```python
from build123d import *

# Parameters (mm, degrees)
BOSS_EXTRUDE1_DEPTH = 10.52068
BOSS_EXTRUDE3_DEPTH = 5.588
SKETCH4_R           = 1.037113256
CUT_EXTRUDE1_DEPTH  = 5.588
SKETCH5_R           = 0.970454713
CUT_EXTRUDE2_DEPTH  = 10.52068


with BuildPart() as part:
    # Sketch1 → Boss-Extrude1 (new body)
    with BuildSketch(Plane(origin=(0, 0, 0), x_dir=(0, 0, -1), z_dir=(1, 0, 0))):
        with BuildLine():
            Line((0, 0), (0, 5.588000005))
            add(Edge.make_bspline(
                [(0, 5.588000005), (50.799999991, 5.588000023), (101.6, -45.211999941)],
                knots=[0.084768036, 0.084768036, 0.084768036, 0.932448396, 0.932448396, 0.932448396], degree=2))
            Line((101.6, -45.211999941), (101.6, -50.799999941))
            add(Edge.make_bspline(
                [(0, 0), (50.79999999, 2e-08), (101.6, -50.799999941)],
                knots=[0.084768036, 0.084768036, 0.084768036, 0.932448396, 0.932448396, 0.932448396], degree=2))
        make_face()
    extrude(amount=BOSS_EXTRUDE1_DEPTH)

    # Sketch2 → Boss-Extrude3 (add)
    with BuildSketch(Plane(origin=(0, 0, 0), x_dir=(1, 0, 0), z_dir=(0, 1, 0))):
        Polygon((0, 0), (10.52068, 0), (5.26034, -7.512544086), align=None)
    extrude(amount=BOSS_EXTRUDE3_DEPTH)

    # Sketch4 → Cut-Extrude1 (cut)
    with BuildSketch(Plane(origin=(0, 5.588000005, 0), x_dir=(1, 0, 0), z_dir=(0, 1, 0))):
        with Locations((5.26034, -2.137251975)):
            Circle(SKETCH4_R)
    extrude(amount=-CUT_EXTRUDE1_DEPTH, mode=Mode.SUBTRACT)

    # Sketch5 → Cut-Extrude2 (cut)
    with BuildSketch(Plane.ZY):
        with Locations((-98.825997746, -45.21199994)):
            Circle(SKETCH5_R)
    extrude(amount=-CUT_EXTRUDE2_DEPTH, mode=Mode.SUBTRACT)


solid = part.part
```
Input: part model. Units: mm. Frame: model coordinates. A direction names the side the tool comes from. Coordinates: 2 decimals unless noted, no trailing zeros.
1) Pin query (flat end, axial travel): pin 1 Ø6 at (x, y) = (6, -36) entering from -Z; pin 2 Ø4 at (x, y) = (6.5, -40) entering from +Z; pin 3 Ø1 at (x, z) = (4.5, -62) entering from +Y. Return the tip coordinate at first contact, or that it passes through.
2) Set-up query: faces 4 (the flat face through (5, 0, 4)), 5 (the flat face through (2.67, 2.75, 3.81)). Return all of +Z, -Z, +X, -X, +Y, -Y with unobstructed straight access to the full face (end or side cutting, diameter ignored); none if empty.
3) Material intervals for line 1 along Y through (x, z) = (0.5, -15); line 2 along Z through (x, y) = (5.25, -29); line 3 along Y through (x, z) = (3, -54), sorted ascending.
4) Mould query, pull axis Z, two halves, no side actions, for faces 1 (the cylindrical face through (5.739, 2.833, 3.057)), 2 (the flat face through (7.93, 2.75, 3.7)), 3 (the flat face through (0, -12, -51)). Classes: pulls with the +Z half, pulls with the -Z half, needs draft (parallel to the pull), parting line crosses it, or undercut.
Check result:
1. pin 1: stops at z = -95.19
1. pin 2: stops at z = -87.87
1. pin 3: stops at y = -13.03
2. face 4: +Z, +X, -X, -Y
2. face 5: +Z, -X, +Y, -Y
3. line 1: y = -1.11 to 4.48
3. line 2: z = -83.83 to -76.76
3. line 3: y = -14.35 to -8.76
4. face 1: undercut
4. face 2: pulls with the +Z half
4. face 3: needs draft
